The drawing under review shows one solid part. Ordinate dimensions are in mm from its lowest x, y, z. A direction names the side the tool comes from. Coordinates: 2 decimals unless noted, no trailing zeros. Write each loop counter-clockwise with the first axis right and the second up, starting at its lowest first coordinate (ties: lowest second). Pieces come first, ordered by that corner, then holes. Notation, with made-up numbers: M -12.5,-14.75 L 17.5,-14.75 A32 ccw 17.5,23.25 Z; hole C 32,-20 d10. An arc over 180 degrees is marked long. Write item = value, one per line.
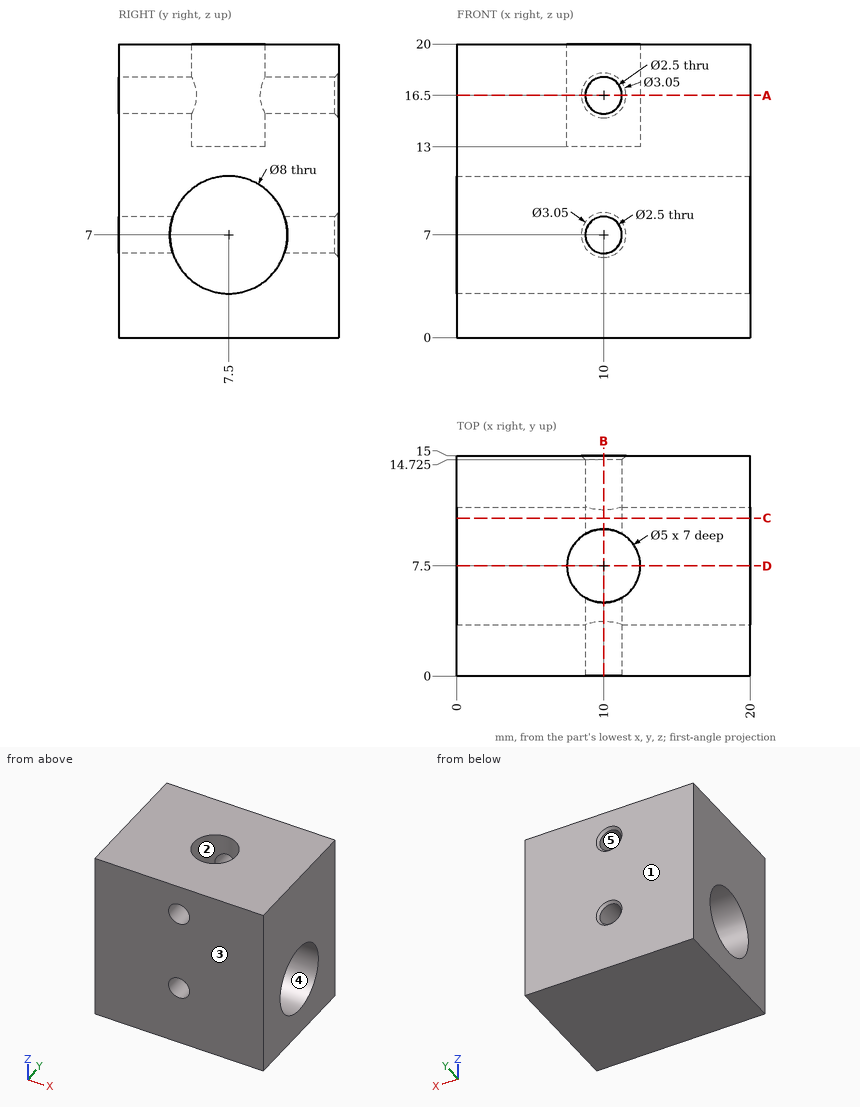
Q1. Consider section D-D, the plane y = 7.5. State the section outline as (x, z) points, and give its area (3 significant figures).
Check result:
outline = M 0,0 L 20,0 L 20,3 L 0,3 Z; M 0,11 L 20,11 L 20,20 L 12.5,20 L 12.5,13 L 7.5,13 L 7.5,20 L 0,20 Z
area = 205 mm²
Q2. The part is to be moulded in two halves that separate along Y. For the marked faces 3, 4 and 5, say which applies: +Y half, -Y half, draft (parallel to the pull), parting line (faces both ways), or undercut.
Check result:
face_3 = -Y half
face_4 = undercut
face_5 = draft
Q3. Consider section A-A, the plane z = 16.5. State the section outline as (x, y) points (3 decimals), and give its area (3 significant figures).
Check result:
outline = M 0,0 L 8.75,0 L 8.75,5.335 A2.5 cw 8.75,9.665 L 8.75,14.725 L 8.475,15 L 0,15 Z; M 11.25,0 L 20,0 L 20,15 L 11.525,15 L 11.25,14.725 L 11.25,9.665 A2.5 cw 11.25,5.335 Z
area = 255 mm²
Q4. Machinability: for the marked faces 1 and 2, which of the approach directions +Z, -Z, +X, -X, +Y, -Y give a long, thin tool a straight path to every point of the face, cutting with its end or side? Answer none if there is none.
Check result:
face_1 = +Z, -Z, +X, -X, +Y
face_2 = +Z
Q5. Consider section B-B, the plane x = 10. State the section outline as (y, z) points (3 decimals), and give its area (3 significant figures).
Check result:
outline = M 0,0 L 15,0 L 15,5.475 L 14.725,5.75 L 11.3,5.75 A4 cw 3.7,5.75 L 0,5.75 Z; M 0,8.25 L 3.7,8.25 A4 cw 11.3,8.25 L 14.725,8.25 L 15,8.525 L 15,14.975 L 14.725,15.25 L 10,15.25 L 10,13 L 5,13 L 5,15.25 L 0,15.25 Z; M 0,17.75 L 5,17.75 L 5,20 L 0,20 Z; M 10,17.75 L 14.725,17.75 L 15,18.025 L 15,20 L 10,20 Z
area = 172 mm²
Q6. Wall thickness on line 1 (X direction, y = 4.2, z = 16.5); line 2 (Z direction, x = 17.5, y = 10.75); line 3 (Z direction, x = 12.25, y = 4.5): over which ranges is each line inside the solid? List them lowest first.
Check result:
line_1 = 0 to 8.75, 11.25 to 20
line_2 = 0 to 4.67, 9.33 to 20
line_3 = 0 to 4.35, 9.65 to 20
Q7. Consider section C-C, the plane y = 10.75. State the section outline as (x, z) points.
Check result:
outline = M 0,0 L 20,0 L 20,4.67 L 0,4.67 Z; M 0,9.33 L 20,9.33 L 20,20 L 0,20 Z; hole C 10,16.5 d2.5
Q8. For P1, Ø3, axis at x = 10, z = 16.5, coming from the +Y side (3 decimals); P2, Ø2.5, axis at x = 9, y = 8, coming from the +Z side; P3, Ø1.5, axis at x = 10, z = 7, coming from the -Y side, all flat-tipped, find the tip position at first contact; note any pin that passes through.
Check result:
P1 = 14.975
P2 = 13
P3 = through
